from build123d import *

# Parameters (mm, degrees)
PAD_DEPTH       = 15
SKETCH002_R     = 67
POCKET_DEPTH    = 13.5
POCKET001_DEPTH = 13.5
PAD001_DEPTH    = 35
PAD002_DEPTH    = 35


with BuildPart() as part:
    # Sketch001 → Pad (new body)
    with BuildSketch(Plane.XY):
        with BuildLine():
            ThreePointArc((67.082039, 20), (42.17208, 55.870526), (0.847707, 69.994867))
            Line((0.847707, 69.994867), (-65, 70.792348))
            ThreePointArc((-65, 70.792348), (-87.960697, 33.627781), (-44.368352, 30.780665))
            ThreePointArc((51.749002, 15.428571), (8.517053, 53.324102), (-44.368352, 30.780665))
            ThreePointArc((51.749002, 15.428571), (61.701235, 10.047767), (67.082039, 20))
        make_face()
    extrude(amount=PAD_DEPTH)

    # Sketch002 → Pocket (cut)
    with BuildSketch(Plane(origin=(0, 0, 0), x_dir=(1, 0, 0), z_dir=(0, 0, -1))):
        Circle(SKETCH002_R)
    extrude(amount=-POCKET_DEPTH, mode=Mode.SUBTRACT)

    # Sketch003 → Pocket001 (cut)
    with BuildSketch(Plane(origin=(0, 0, 0), x_dir=(1, 0, 0), z_dir=(0, 0, -1))):
        Polygon((-152.534362, -68.852256), (0.811393, -66.995087), (-35.4631, 35.7409), align=None)
    extrude(amount=-POCKET001_DEPTH, mode=Mode.SUBTRACT)

    # Sketch005 → Pad001 (new body)
    with BuildSketch(Plane.XY.offset(15)):
        Polygon((37.550363, 56.878996), (41.718314, 61.195035), (59.701809, 43.828576), (55.533858, 39.512537), align=None)
    extrude(amount=-PAD001_DEPTH)

    # Sketch006 → Pad002 (new body)
    with BuildSketch(Plane.XY.offset(15)):
        Polygon((-37.856891, 67.463398), (-39.909012, 73.101554), (-16.416696, 81.652057), (-11.134654, 67.139765), align=None)
    extrude(amount=-PAD002_DEPTH)


solid = part.part
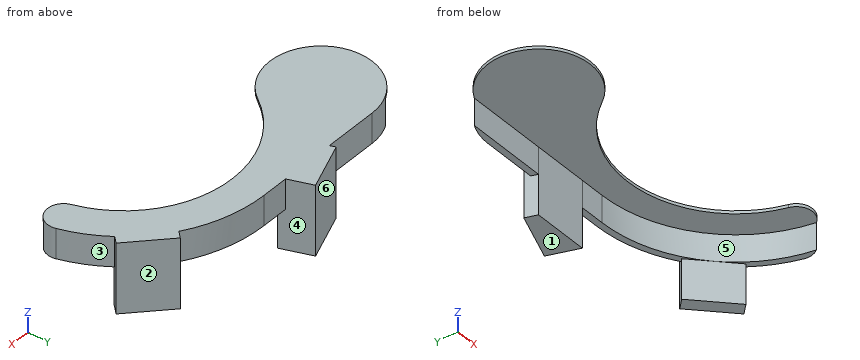
Could you check a few things on this model? Use its own coordinates, in mm. Face numbers are marked on the shaded views. A direction names the side the tool comes from. Give positions to 0.01 mm unless a question says otherwise; leave off trailing zeros. Order: outer loops, then holes, each group sorted by start corner. A loop starts at its lowest first (then second) coordinate and runs counter-clockwise, first axis right, second up. Notation, with made-up numbers: (48.25, 85.25) -> (82.25, 85.25) arc R31 cw to (82.25, 114.25) -> close; hole circle Ø5 at (-3, -13). An arc over 180 degrees is marked (long way). Return JSON: item names as keys, results as strings.
1. Imagine slicing it at C-C on y = 35. List the corners of the cut face in (x, z) for me, then the cut area to 3 significant figures.
Answer list:
{"outline": "(-88.62, 13.5) -> (-41.12, 13.5) -> (-41.12, 15) -> (-88.62, 15) -> close; (41.12, 13.5) -> (57.13, 13.5) -> (57.13, 0) -> (60.62, 0) -> (60.62, 15) -> (41.12, 15) -> close", "area": "148 mm2"}
2. Thinking about a two-plate mould opening in Y: for the marked faces 1, 2 and 3, which applies, pulls with the +Y half, pulls with the -Y half, needs draft (parallel to the pull), parting line crosses it, or undercut?
Answer list:
{"face 1": "needs draft", "face 2": "pulls with the +Y half", "face 3": "undercut"}
3. I need wall thicknesses on line 1 (Z direction, x = -68, y = 48.5); line 2 (X direction, y = 18.5, z = 10); line 3 (X direction, y = 57.5, z = 9.5). Which ranges of each line are inside material? Lowest first, please. Write a range as from..to.
Answer list:
{"line 1": "z = 13.5..15", "line 2": "x = 64.4..67.38", "line 3": "x = 34.39..45.54"}
4. Imagine slicing it at B-B on z = -9. List the corners of the cut face in (x, y) for me, then the cut area to 3 significant figures.
Answer list:
{"outline": "(-39.91, 73.1) -> (-37.86, 67.46) -> (-11.13, 67.14) -> (-16.42, 81.65) -> close; (37.55, 56.88) -> (55.53, 39.51) -> (59.7, 43.83) -> (41.72, 61.2) -> close", "area": "418 mm2"}
5. Imagine slicing it at D-D on x = -28.5. List the corners of the cut face in (y, z) for me.
Answer list:
{"outline": "(45.87, 13.5) -> (67.35, 13.5) -> (67.35, -20) -> (77.25, -20) -> (77.25, 15) -> (45.87, 15) -> close"}
6. Imagine slicing it at A-A on z = 2.5. List the corners of the cut face in (x, y) for me, then the cut area to 3 significant figures.
Answer list:
{"outline": "(-77.03, 67.94) -> (0.81, 67) arc R67 cw to (65.76, 12.84) arc R8 ccw to (67.08, 20) arc R70 ccw to (56.84, 40.86) -> (59.7, 43.83) -> (41.72, 61.2) -> (38.85, 58.23) arc R70 ccw to (0.85, 69.99) -> (-12.23, 70.15) -> (-16.42, 81.65) -> (-39.91, 73.1) -> (-38.95, 70.48) -> (-65, 70.79) arc R25.49 ccw to start", "area": "769 mm2"}
7. For pin 1 Ø1 at (x, z) = (-56, 8.5) entering from -Y; pin 2 Ø6.5 at (x, y) = (54.5, 39) entering from -Z; pin 3 Ø6.5 at (x, y) = (22, 60) entering from -Z; pin 4 Ø12 at (x, z) = (-10.5, -7) entering from -Y, each with a flat end and sliding along its axis, tell me the tip position at first contact or that it passes through.
Answer list:
{"pin 1": "stops at y = 67.68", "pin 2": "stops at z = -20", "pin 3": "stops at z = 0", "pin 4": "stops at y = 67.14"}
8. On a 3-axis mill with a long thin cutter (end or side, diameter ignored), from which of +Z, -Z, +X, -X, +Y, -Y can I reach the whole of each face in a straight line? I mean the marked faces 4, 5 and 6. Say none if no direction works.
Answer list:
{"face 4": "-Z, +X, +Y", "face 5": "-Z, -X, -Y", "face 6": "+Z, -Z, -X, +Y"}
